The listing builds one solid part. Answer for the finished solid, in the listing's coordinates (mm). Round coordinates to 2 decimals unless told otherwise and drop trailing zeros. Write each loop counter-clockwise with the first axis right and the second up, starting at its lowest first coordinate (ties: lowest second). Pieces come first, ordered by that corner, then holes. Notation, with made-up numbers: (66.5, 65.5) - (117.5, 65.5) arc R8 cw to (117.5, 76.5) - close; hole circle Ø5 at (-35, -11.75). An arc over 180 degrees is marked (long way). Answer in a Markdown table with one row per item.
from build123d import *

# Parameters (mm, degrees)
BOSS_EXTRUDE1_DEPTH      = 609.6
BOSS_EXTRUDE1_DEPTH_BACK = 609.6
SKETCH5_R                = 5.334
CUT_EXTRUDE1_DEPTH       = 16.875
SKETCH6_R                = 5.334
CUT_EXTRUDE2_DEPTH       = 16.875
LPATTERN1_COUNT          = 48
LPATTERN1_PITCH          = 25.4
SKETCH7_W                = 635
SKETCH7_H                = 31.75
CUT_EXTRUDE3_DEPTH       = 70
SKETCH8_R                = 5.334
SKETCH8_W                = 25.4
SKETCH8_H                = 4.1148
CUT_EXTRUDE4_DEPTH       = 70


with BuildPart() as part:
    # Sketch4 → Boss-Extrude1 (new body, two sides)
    with BuildSketch(Plane(origin=(0, 0, 0), x_dir=(0, 0, -1), z_dir=(1, 0, 0))) as boss_extrude1_sk:
        with BuildLine():
            Line((-15.875, -13.1318), (11.7602, -13.1318))
            ThreePointArc((11.7602, -13.1318), (12.730067661, -12.730067661), (13.1318, -11.7602))
            Line((13.1318, -11.7602), (13.1318, 15.875))
            Line((13.1318, 15.875), (15.875, 15.875))
            Line((15.875, 15.875), (15.875, -11.7602))
            ThreePointArc((15.875, -11.7602), (14.669802983, -14.669802983), (11.7602, -15.875))
            Line((11.7602, -15.875), (-15.875, -15.875))
            Line((-15.875, -15.875), (-15.875, -13.1318))
        make_face()
    extrude(amount=BOSS_EXTRUDE1_DEPTH)
    extrude(boss_extrude1_sk.sketch, amount=-BOSS_EXTRUDE1_DEPTH_BACK)

    # Sketch5 → Cut-Extrude1 (cut, through all)
    with BuildSketch(Plane.XY):
        with Locations((596.9, 0)):
            Circle(SKETCH5_R)
    cut_extrude1 = extrude(amount=-CUT_EXTRUDE1_DEPTH, mode=Mode.SUBTRACT)

    # Sketch6 → Cut-Extrude2 (cut, through all)
    with BuildSketch(Plane(origin=(0, 0, 0), x_dir=(1, 0, 0), z_dir=(0, 1, 0))):
        with Locations((596.9, 0)):
            Circle(SKETCH6_R)
    cut_extrude2 = extrude(amount=-CUT_EXTRUDE2_DEPTH, mode=Mode.SUBTRACT)

    # LPattern1: Cut-Extrude1, Cut-Extrude2 ×48
    with Locations(*[(-i * LPATTERN1_PITCH, 0, 0) for i in range(1, LPATTERN1_COUNT)]):
        add(cut_extrude1, mode=Mode.SUBTRACT)
        add(cut_extrude2, mode=Mode.SUBTRACT)

    # Sketch7 → Cut-Extrude3 (cut)
    with BuildSketch(Plane(origin=(0, 0, -15.875), x_dir=(-1, 0, 0), z_dir=(0, 0, -1))):
        with Locations((-292.1, 0)):
            Rectangle(SKETCH7_W, SKETCH7_H)
    extrude(amount=-CUT_EXTRUDE3_DEPTH, mode=Mode.SUBTRACT)

    # Sketch8 → Cut-Extrude4 (cut)
    with BuildSketch(Plane(origin=(0, 0, -15.875), x_dir=(-1, 0, 0), z_dir=(0, 0, -1))):
        Polygon((50.8, 15.875), (25.4, 15.875), (25.4, -11.7602), (50.8, -11.7602), (50.8, 0), align=None)
        with Locations((38.1, 0)):
            Circle(SKETCH8_R, mode=Mode.SUBTRACT)
        with Locations((38.1, -13.8176)):
            Rectangle(SKETCH8_W, SKETCH8_H)
    extrude(amount=-CUT_EXTRUDE4_DEPTH, mode=Mode.SUBTRACT)


solid = part.part
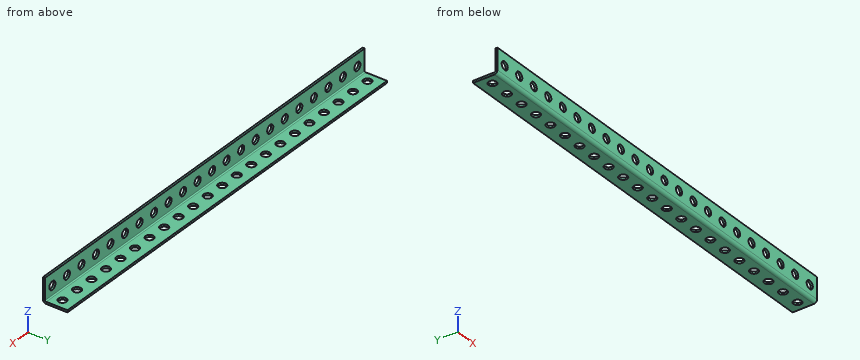
(1) Find the intervals of material crossed by line 1 (Z direction, x = -364, y = -8.5) (3 decimals); line 2 (Y direction, x = -292, z = -14) (3 decimals), in increasing order.
Checked values:
| item | result |
|---|---|
| line 1 | z = -15.875 to -13.132 |
| line 2 | y = -15.212 to -5.333, 5.333 to 15.875 |
(2) Section B-B (z = 0) is taken. State how many separate pieces and enclosed holes the cut face has, and give its area (3 significant figures).
Checked values:
| item | result |
|---|---|
| separate pieces | 23 |
| enclosed holes | 0 |
| area | 889 mm2 |
(3) Flat-ended cylindrical pins translate along their axes: pin 1 (12.5 mm diameter, centred on x = -342.9, z = 0, fed in from +Y); pin 2 (12.5 mm diameter, centred on x = -444.5, y = 0, fed in from +Z). Find the tip coordinate at first contact, or state that the pin passes through.
Checked values:
| item | result |
|---|---|
| pin 1 | stops at y = -13.13 |
| pin 2 | stops at z = -13.13 |
(4) Section A-A (x = -393.7) is taken. Give the vertices of the cut face in (y, z) (3 decimals), and give its area (3 significant figures).
Checked values:
| item | result |
|---|---|
| outline | (-15.875, -11.76) arc R4.115 ccw to (-11.76, -15.875) - (-5.334, -15.875) - (-5.334, -13.132) - (-11.76, -13.132) arc R1.372 cw to (-13.132, -11.76) - (-13.132, -5.334) - (-15.875, -5.334) - close; (-15.875, 5.334) - (-13.132, 5.334) - (-13.132, 15.875) - (-15.875, 15.875) - close; (5.334, -15.875) - (15.875, -15.875) - (15.875, -13.132) - (5.334, -13.132) - close |
| area | 105 mm2 |
